from build123d import *

# Parameters (mm, degrees)
F_98MM_6ID_CENTERING_RING_SKETCH_R = 53.34
CENTERING_RING_EXTRUDE_DEPTH       = 1.905
CENTERING_RING_EXTRUDE_DEPTH_BACK  = 1.905
CUT_EXTRUDE3_DEPTH                 = 4.81
CIRPATTERN1_COUNT                  = 6
CIRPATTERN1_ANGLE                  = 25
SKETCH5_R                          = 3.048
SKETCH5_R_2                        = 2.54
SKETCH5_R_3                        = 7.9375
CUT_EXTRUDE4_DEPTH                 = 3.81


with BuildPart() as part:
    # 98mm - 6ID centering ring sketch → Centering Ring Extrude (new body, two sides)
    with BuildSketch(Plane(origin=(0, 0, 0), x_dir=(1, 0, 0), z_dir=(0, 1, 0))) as centering_ring_extrude_sk:
        with BuildLine():
            Line((56.425744124, 3.175), (99.009105516, 3.175))
            ThreePointArc((99.009105516, 3.175), (70.045997744, 70.045997744), (3.175, 99.009105516))
            Line((3.175, 99.009105516), (3.175, 56.425744124))
            ThreePointArc((3.175, 56.425744124), (0, 56.515), (-3.175, 56.425744124))
            Line((-3.175, 56.425744124), (-3.175, 99.009105516))
            ThreePointArc((-3.175, 99.009105516), (-70.045997744, 70.045997744), (-99.009105516, 3.175))
            Line((-99.009105516, 3.175), (-56.425744124, 3.175))
            ThreePointArc((-56.425744124, 3.175), (-56.515, 0), (-56.425744124, -3.175))
            Line((-56.425744124, -3.175), (-99.009105516, -3.175))
            ThreePointArc((-99.009105516, -3.175), (-70.045997744, -70.045997744), (-3.175, -99.009105516))
            Line((-3.175, -99.009105516), (-3.175, -56.425744124))
            ThreePointArc((-3.175, -56.425744124), (0, -56.515), (3.175, -56.425744124))
            Line((3.175, -56.425744124), (3.175, -99.009105516))
            ThreePointArc((3.175, -99.009105516), (70.045997744, -70.045997744), (99.009105516, -3.175))
            Line((99.009105516, -3.175), (56.425744124, -3.175))
            ThreePointArc((56.425744124, -3.175), (56.515, 0), (56.425744124, 3.175))
        make_face()
        Circle(F_98MM_6ID_CENTERING_RING_SKETCH_R, mode=Mode.SUBTRACT)
        with BuildLine():
            ThreePointArc((99.06, 0), (99.047275562, 1.587703943), (99.009105516, 3.175))
            Line((99.009105516, 3.175), (56.425744124, 3.175))
            ThreePointArc((56.425744124, 3.175), (56.515, 0), (56.425744124, -3.175))
            Line((56.425744124, -3.175), (99.009105516, -3.175))
            ThreePointArc((99.009105516, -3.175), (99.047275562, -1.587703943), (99.06, 0))
        make_face()
        with BuildLine():
            Line((3.175, 56.425744124), (3.175, 99.009105516))
            ThreePointArc((3.175, 99.009105516), (0, 99.06), (-3.175, 99.009105516))
            Line((-3.175, 99.009105516), (-3.175, 56.425744124))
            ThreePointArc((-3.175, 56.425744124), (0, 56.515), (3.175, 56.425744124))
        make_face()
        with BuildLine():
            Line((-56.425744124, 3.175), (-99.009105516, 3.175))
            ThreePointArc((-99.009105516, 3.175), (-99.06, 0), (-99.009105516, -3.175))
            Line((-99.009105516, -3.175), (-56.425744124, -3.175))
            ThreePointArc((-56.425744124, -3.175), (-56.515, 0), (-56.425744124, 3.175))
        make_face()
        with BuildLine():
            ThreePointArc((-3.175, -99.009105516), (0, -99.06), (3.175, -99.009105516))
            Line((3.175, -99.009105516), (3.175, -56.425744124))
            ThreePointArc((3.175, -56.425744124), (0, -56.515), (-3.175, -56.425744124))
            Line((-3.175, -56.425744124), (-3.175, -99.009105516))
        make_face()
    extrude(amount=CENTERING_RING_EXTRUDE_DEPTH)
    extrude(centering_ring_extrude_sk.sketch, amount=-CENTERING_RING_EXTRUDE_DEPTH_BACK)

    # Sketch3 → Cut-Extrude3 (cut, through all)
    with BuildSketch(Plane(origin=(0, 1.905, 0), x_dir=(1, 0, 0), z_dir=(0, 1, 0))):
        with BuildLine():
            Line((-22.283651443, 96.521098618), (-19.141085214, 82.909148813))
            ThreePointArc((-19.141085214, 82.909148813), (-18.41684675, 83.073027246), (-17.691205772, 83.230579346))
            Line((-17.691205772, 83.230579346), (-20.595732092, 96.895301329))
            ThreePointArc((-20.595732092, 96.895301329), (-21.440508157, 96.711882465), (-22.283651443, 96.521098618))
        make_face()
    cut_extrude3 = extrude(amount=-CUT_EXTRUDE3_DEPTH, mode=Mode.SUBTRACT)

    # CirPattern1: Cut-Extrude3 ×6 about axis
    cirpattern1_axis = Axis((0, 0, 0), (0, -1, 0))
    for i in range(1, CIRPATTERN1_COUNT):
        add(cut_extrude3.rotate(cirpattern1_axis, i * CIRPATTERN1_ANGLE / (CIRPATTERN1_COUNT - 1)), mode=Mode.SUBTRACT)

    # Sketch5 → Cut-Extrude4 (cut)
    with BuildSketch(Plane.XZ.offset(1.905)):
        with Locations((-62.419385775, 43.70652445)):
            Circle(SKETCH5_R)
        with Locations((-44.082374272, 52.535327909)):
            Circle(SKETCH5_R_2)
        with Locations((44.082374272, 52.535327909)):
            Circle(SKETCH5_R_2)
        with Locations((62.419385775, 43.70652445)):
            Circle(SKETCH5_R)
        with Locations((62.419385775, -43.70652445)):
            Circle(SKETCH5_R)
        with Locations((44.082374272, -52.535327909)):
            Circle(SKETCH5_R_2)
        with Locations((-44.082374272, -52.535327909)):
            Circle(SKETCH5_R_2)
        with Locations((-62.419385775, -43.70652445)):
            Circle(SKETCH5_R)
        with Locations((0, 74.75474)):
            Circle(SKETCH5_R_3)
    extrude(amount=-CUT_EXTRUDE4_DEPTH, mode=Mode.SUBTRACT)


solid = part.part
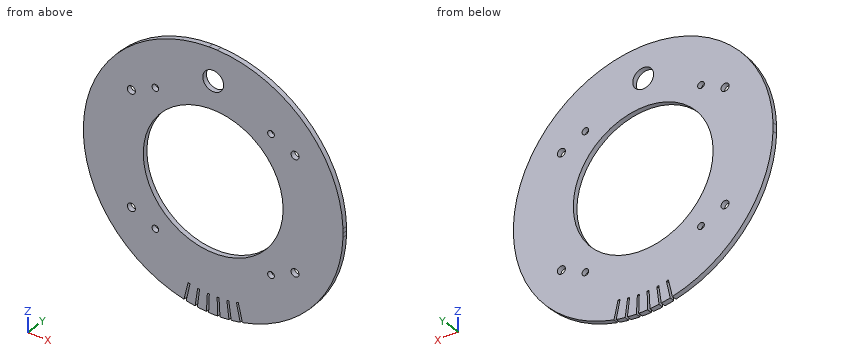
The listing builds one solid part. Answer for the finished solid, in the listing's coordinates (mm). Coordinates: 2 decimals unless noted, no trailing zeros. Order: outer loops, then holes, each group sorted by start corner. A loop starts at its lowest first (then second) coordinate and runs counter-clockwise, first axis right, second up.
Q1. A cutting plane is placed at B-B, the plane z = 19. Write down the section's boundary in (x, y) (3 decimals).
Q2. A cutting plane is placed at A-A, the plane x = 0. Write down the section's boundary in (y, z) (3 decimals), and give its area (3 significant figures).
Q3. Given P1, Ø1.5, axis at y = -1.5, z = 45.5, coming from the -X side; P2, Ø2, axis at y = -1.5, z = 25, coming from the -X side; P3, Ø3.5, axis at x = 62.42, z = -43.71, coming from the -Y side; P4, Ø2, axis at x = -6.5, y = -1, coming from the -Z side, each flat-ended and moving along its own axis, determine where each tip first touches the part or whether it passes through.
Q4. Consider line 1 (Z direction, x = 0, y = -1.1); line 2 (Z direction, x = 46, y = -0.75); line 3 (Z direction, x = -44, y = 0.05). Determine where each line is inside the solid, lowest interval first.
Q5. A cutting plane is placed at C-C, the plane z = -31. Write down the section's boundary in (x, y) (3 decimals).
Q6. A cutting plane is placed at D-D, the plane y = 0.05. State how many separate pieces and enclosed holes the cut face has, and give its area (3 significant figures).
Answers follow:
1. outline: (-97.221, -1.905) - (-49.841, -1.905) - (-49.841, 1.905) - (-97.221, 1.905) - close; (49.841, -1.905) - (97.221, -1.905) - (97.221, 1.905) - (49.841, 1.905) - close
2. outline: (-1.905, -99.06) - (1.905, -99.06) - (1.905, -53.34) - (-1.905, -53.34) - close; (-1.905, 53.34) - (1.905, 53.34) - (1.905, 66.817) - (-1.905, 66.817) - close; (-1.905, 82.692) - (1.905, 82.692) - (1.905, 99.06) - (-1.905, 99.06) - close
2. area: 288 mm2
3. P1: stops at x = -88.38
3. P2: stops at x = -96.11
3. P3: passes through
3. P4: stops at z = -98.91
4. line 1: z = -99.06 to -53.34, 53.34 to 66.82, 82.69 to 99.06
4. line 2: z = -87.73 to -54.2, -50.87 to -27, 27 to 50.87, 54.2 to 87.73
4. line 3: z = -88.75 to -55.07, -50 to -30.15, 30.15 to 50, 55.07 to 88.75
5. outline: (-94.084, -1.905) - (-43.407, -1.905) - (-43.407, 1.905) - (-94.084, 1.905) - close; (43.407, -1.905) - (94.084, -1.905) - (94.084, 1.905) - (43.407, 1.905) - close
6. separate pieces: 1
6. enclosed holes: 10
6. area: 21,400 mm2
